Autodesk Inventor part; units mm, degrees
ref_plane "YZ Plane" through (0, 0, 0) normal (1, 0, 0) x (0, 1, 0)
ref_plane "XZ Plane" through (0, 0, 0) normal (0, 1, 0) x (-1, 0, 0)
ref_plane "XY Plane" through (0, 0, 0) normal (0, 0, 1) x (1, 0, 0)
sketch "草图1" plane through (0, 0, 0) normal (0, 1, 0) x (-1, 0, 0)
  line L0 (110.5, 55.5) -> (-110.5, 55.5)
  line L1 (-110.5, 55.5) -> (-110.5, -55.5)
  line L2 (-110.5, -55.5) -> (110.5, -55.5)
  line L3 (110.5, -55.5) -> (110.5, 55.5)
  line L4 (0, 7.5575) -> (0, -11)
  line L5 (8.5019, 0) -> (-7, 0)
  point P0 (0, 0)
  point P1 (0, 0)
  point P2 (0, 0)
  dimension "d0" = 221
  dimension "d1" = 111
extrude "拉伸1" add sketch "草图1" along normal blind 6
fillet "圆角1" radius 10.1 1 edges at (-110.5, 3, -55.5)
sketch "草图2" plane through (0, 6, 0) normal (0, 1, 0) x (1, 0, 0)
  circle A0 centre (-64.5, 9.5) radius 10.05
  line L0 (110.5, 55.5) -> (-100.4, 55.5)
  line L1 (-110.5, 45.4) -> (-110.5, -55.5)
  point P0 (0, 0)
  dimension "d5" = 20.1
  dimension "d6" = 46
  dimension "d7" = 46
extrude "拉伸2" cut sketch "草图2" against normal blind 6
sketch "草图3" plane through (0, 6, 0) normal (0, 1, 0) x (1, 0, 0)
  circle A0 centre (-104.5, 25.5) radius 2.1
  circle A1 centre (-104.5, -25.5) radius 2.1
  line L0 (-110.5, -55.5) -> (-110.5, 55.5)
  line L1 (110.5, -55.5) -> (-110.5, -55.5)
  line L2 (-110.5, 55.5) -> (100.4, 55.5)
  circle A2 centre (104.5, -25.5) radius 2.1
  circle A3 centre (104.5, 25.5) radius 2.1
  line L3 (110.5, -55.5) -> (110.5, 55.5)
  point P0 (0, 0)
  point P1 (0, 0)
  dimension "d10" = 4.2
  dimension "d11" = 4.2
  dimension "d12" = 6
  dimension "d13" = 6
  dimension "d14" = 30
  dimension "d15" = 30
  dimension "d16" = 4.2
  dimension "d17" = 4.2
  dimension "d18" = 30
  dimension "d19" = 6
  dimension "d20" = 30
  dimension "d21" = 6
extrude "拉伸3" cut sketch "草图3" against normal blind 10 contours A2 | A3
sketch "草图4" plane through (0, 6, 0) normal (0, 1, 0) x (1, 0, 0)
  circle A0 centre (104.5, -25.5) radius 2.1
  circle A1 centre (104.5, -25.5) radius 3.6
  circle A2 centre (104.5, 25.5) radius 2.1
  circle A3 centre (104.5, 25.5) radius 3.6
  point P0 (0, 0)
  dimension "d24" = 7.2
  dimension "d25" = 7.2
extrude "拉伸4" cut sketch "草图4" against normal blind 4 contours A0 | A1 | A2 | A3
sketch "草图5" plane through (0, 6, 0) normal (0, 1, 0) x (1, 0, 0)
  circle A0 centre (49.5, -40.5) radius 2.1
  circle A1 centre (-50.5, -40.5) radius 2.1
  line L0 (-110.5, -55.5) -> (110.5, -55.5)
  line L1 (-110.5, 45.4) -> (-110.5, -55.5)
  point P0 (0, 0)
  dimension "d28" = 4.2
  dimension "d29" = 4.2
  dimension "d30" = 15
  dimension "d31" = 15
  dimension "d32" = 60
  dimension "d33" = 100
extrude "拉伸5" cut sketch "草图5" against normal blind 6
sketch "草图6" plane through (0, 6, 0) normal (0, 1, 0) x (1, 0, 0)
  circle A0 centre (49.5, -40.5) radius 2.1
  circle A1 centre (49.5, -40.5) radius 3.6
  circle A2 centre (-50.5, -40.5) radius 2.1
  circle A3 centre (-50.5, -40.5) radius 3.6
  point P0 (0, 0)
  dimension "d36" = 7.2
  dimension "d37" = 7.2
extrude "拉伸6" cut sketch "草图6" against normal blind 4 contours A0 | A1 | A2 | A3
properties part number "底板_C"
Source: CAD feature listing. Evaluate the final solid. Frame: model axes, mm. A direction names the side the tool comes from. Give positions to 0.01 mm unless a question says otherwise; leave off trailing zeros. Write each loop counter-clockwise with the first axis right and the second up, starting at its lowest first coordinate (ties: lowest second). Pieces come first, ordered by that corner, then holes. Notation, with made-up numbers: M 82.25,33 L 113.25,33 A25 cw 113.25,71 Z; hole C -38.75,56.25 d8. An arc over 180 degrees is marked long. Return JSON: item names as keys, results as strings. Group by question number.
1) Cut plane D-D, the plane z = 25.5. Output: boundary loops of the cut face in (x, y).
2) First-contact query: pin 1 Ø5.5 at (x, z) = (104.5, 25.5) entering from -Y; pin 2 Ø2 at (x, z) = (-51.5, 41.5) entering from +Y. Flat tips, straight axial feed; report the tip coordinate or a pass-through.
3) Set-up query: faces 4 (the face through (7, 3, -55.5)), 5 (the face through (-48, 2, 40)). Return all of +Z, -Z, +X, -X, +Y, -Y with unobstructed straight access to the full face (end or side cutting, diameter ignored); none if empty.
4) Cut plane A-A, the plane z = 40.5. Output: boundary loops of the cut face in (x, y), then the cut area to 3 significant figures.
5) Ray query, L1, parallel to X at y = 1.65, z = 40.5; L2, parallel to X at y = 1.85, z = -9.5; L3, parallel to Z at x = 104.5, y = 1.2. Return the intervals inside material, ascending.
6) Cut plane B-B, the plane y = 4.5. Output: boundary loops of the cut face in (x, z), then the cut area to 3 significant figures.
7) Draft query along Z for faces 1 (the face through (-107.46, 3.04, -52.62)), 2 (the face through (51.435, 4.028, 37.464)), 3 (the face through (2, 0, 1)). Return one class per face: released by +Z, released by -Z, zero draft, split by the parting line, or undercut.
8) Cut plane C-C, the plane x = -50.5. Output: boundary loops of the cut face in (y, z), then the cut area to 3 significant figures.
Data:
{
 "1": {"outline": "M -110.5,0 L 102.4,0 L 102.4,2 L 100.9,2 L 100.9,6 L -110.5,6 Z; M 106.6,0 L 110.5,0 L 110.5,6 L 108.1,6 L 108.1,2 L 106.6,2 Z"},
 "2": {"pin 1": "stops at y = 0", "pin 2": "stops at y = 2"},
 "3": {"face 4": "-Z, +X, -X, +Y, -Y", "face 5": "+Y"},
 "4": {"outline": "M -110.5,0 L -52.6,0 L -52.6,2 L -54.1,2 L -54.1,6 L -110.5,6 Z; M -48.4,0 L 47.4,0 L 47.4,2 L 45.9,2 L 45.9,6 L -46.9,6 L -46.9,2 L -48.4,2 Z; M 51.6,0 L 110.5,0 L 110.5,6 L 53.1,6 L 53.1,2 L 51.6,2 Z", "area": "1,250 mm²"},
 "5": {"L1": "x = -110.5 to -52.6, -48.4 to 47.4, 51.6 to 110.5", "L2": "x = -110.5 to -74.55, -54.45 to 110.5", "L3": "z = -55.5 to -27.6, -23.4 to 23.4, 27.6 to 55.5"},
 "6": {"outline": "M -110.5,-45.4 A10.1 ccw -100.4,-55.5 L 110.5,-55.5 L 110.5,55.5 L -110.5,55.5 Z; hole C -64.5,-9.5 d20.1; hole C -50.5,40.5 d7.2; hole C 49.5,40.5 d7.2; hole C 104.5,-25.5 d7.2; hole C 104.5,25.5 d7.2", "area": "24,000 mm²"},
 "7": {"face 1": "released by -Z", "face 2": "undercut", "face 3": "zero draft"},
 "8": {"outline": "M 0,-55.5 L 6,-55.5 L 6,36.9 L 2,36.9 L 2,38.4 L 0,38.4 Z; M 0,42.6 L 2,42.6 L 2,44.1 L 6,44.1 L 6,55.5 L 0,55.5 Z", "area": "629 mm²"}
}
